Source: CAD feature listing. Evaluate the final solid. Frame: model axes, mm. A direction names the side the tool comes from. Round coordinates to 2 decimals unless told otherwise and drop trailing zeros. Write each loop counter-clockwise with the first axis right and the second up, starting at its lowest first coordinate (ties: lowest second). Pieces come first, ordered by that corner, then holes.
from build123d import *

# Parameters (mm, degrees)
SKETCH1_R           = 48.25
BOSS_EXTRUDE1_DEPTH = 27.7
SKETCH2_R           = 29.5
BOSS_EXTRUDE2_DEPTH = 6.6
SKETCH3_R           = 29
BOSS_EXTRUDE3_DEPTH = 8
SKETCH4_R           = 3.924903364
CUT_EXTRUDE1_DEPTH  = 8
SKETCH6_W           = 13.813607538
SKETCH6_H           = 65.464487898
SKETCH6_W_2         = 19.669375951
SKETCH6_H_2         = 76.725581
CUT_EXTRUDE2_DEPTH  = 39


with BuildPart() as part:
    # Sketch1 → Boss-Extrude1 (new body)
    with BuildSketch(Plane.XY):
        Circle(SKETCH1_R)
    extrude(amount=-BOSS_EXTRUDE1_DEPTH)

    # Sketch2 → Boss-Extrude2 (add)
    with BuildSketch(Plane.XY):
        Circle(SKETCH2_R)
    extrude(amount=BOSS_EXTRUDE2_DEPTH)

    # Sketch3 → Boss-Extrude3 (add)
    with BuildSketch(Plane(origin=(0, 0, -27.7), x_dir=(-1, 0, 0), z_dir=(0, 0, -1))):
        Circle(SKETCH3_R)
    extrude(amount=BOSS_EXTRUDE3_DEPTH)

    # Sketch4 → Cut-Extrude1 (cut)
    with BuildSketch(Plane.XY.offset(6.6)):
        Circle(SKETCH4_R)
    extrude(amount=-CUT_EXTRUDE1_DEPTH, mode=Mode.SUBTRACT)

    # Sketch6 → Cut-Extrude2 (cut)
    with BuildSketch(Plane.XY):
        with Locations((-53.156803769, 0.938424425)):
            Rectangle(SKETCH6_W, SKETCH6_H)
        with Locations((56.084687976, -0.187684885)):
            Rectangle(SKETCH6_W_2, SKETCH6_H_2)
    extrude(amount=-CUT_EXTRUDE2_DEPTH, mode=Mode.SUBTRACT)


solid = part.part
1) Section query D-D on x = 23. Return the cut outline in (y, z).
Taken from the geometry:
outline: (-42.42, -27.7) - (-17.66, -27.7) - (-17.66, -35.7) - (17.66, -35.7) - (17.66, -27.7) - (42.42, -27.7) - (42.42, 0) - (18.47, 0) - (18.47, 6.6) - (-18.47, 6.6) - (-18.47, 0) - (-42.42, 0) - close
2) Section query A-A on x = 0. Return the cut outline in (y, z).
Taken from the geometry:
outline: (-48.25, -27.7) - (-29, -27.7) - (-29, -35.7) - (29, -35.7) - (29, -27.7) - (48.25, -27.7) - (48.25, 0) - (29.5, 0) - (29.5, 6.6) - (3.92, 6.6) - (3.92, -1.4) - (-3.92, -1.4) - (-3.92, 6.6) - (-29.5, 6.6) - (-29.5, 0) - (-48.25, 0) - close
3) Contact query for flat-ended pins moving along their axis: P1, Ø4, axis at x = 10, z = -1, coming from the -Y side; P2, Ø6.5, axis at x = -1, y = 1, coming from the +Z side; P3, Ø3, axis at y = 28.5, z = -17, coming from the +X side; P4, Ø6, axis at x = -10, z = -22, coming from the +Y side. Output: stop coordinate, or through.
Taken from the geometry:
P1: stops at y = -47.58
P2: stops at z = 6.6
P3: stops at x = 39.99
P4: stops at y = 47.74
4) Pull-direction query (Y, two-part tool) for faces 1 (the face through (46.25, 0, -14)), 2 (the face through (0.866, 48.242, -13.656)), 3 (the face through (28.14, 8.86, 3.25)), 4 (the face through (3.744, 1.179, 2.656)); classes: released by +Y, released by -Y, zero draft, split by the parting line, or undercut.
Taken from the geometry:
face 1: zero draft
face 2: released by +Y
face 3: split by the parting line
face 4: undercut
5) Material intervals for line 1 (Y direction, x = 0, z = 3); line 2 (Z direction, x = -23, y = -38.5); line 3 (Y direction, x = -6.5, z = -19), sorted ascending.
Taken from the geometry:
line 1: y = -29.5 to -3.92, 3.92 to 29.5
line 2: z = -27.7 to 0
line 3: y = -47.81 to 47.81
6) Reachability of faces 5 (the face through (-21, -21, -27.7)), 6 (the face through (0, 0, -35.7)), 7 (the face through (0, 0, -1.4)) from +Z, -Z, +X, -X, +Y, -Y: full face, straight path, thin tool, end or side. Return the list, or none.
Taken from the geometry:
face 5: -Z
face 6: -Z, +X, -X, +Y, -Y
face 7: +Z
7) Section query C-C on z = -4.5. Return the cut outline in (x, y).
Taken from the geometry:
outline: (-46.25, -13.75) arc R48.25 ccw to (46.25, -13.75) - (46.25, 13.75) arc R48.25 ccw to (-46.25, 13.75) - close
8) Section query B-B on y = -1.5. Return the cut outline in (x, z), then the cut area to 3 significant figures.
Taken from the geometry:
outline: (-46.25, -27.7) - (-28.96, -27.7) - (-28.96, -35.7) - (28.96, -35.7) - (28.96, -27.7) - (46.25, -27.7) - (46.25, 0) - (29.46, 0) - (29.46, 6.6) - (3.63, 6.6) - (3.63, -1.4) - (-3.63, -1.4) - (-3.63, 6.6) - (-29.46, 6.6) - (-29.46, 0) - (-46.25, 0) - close
area: 3,360 mm2
